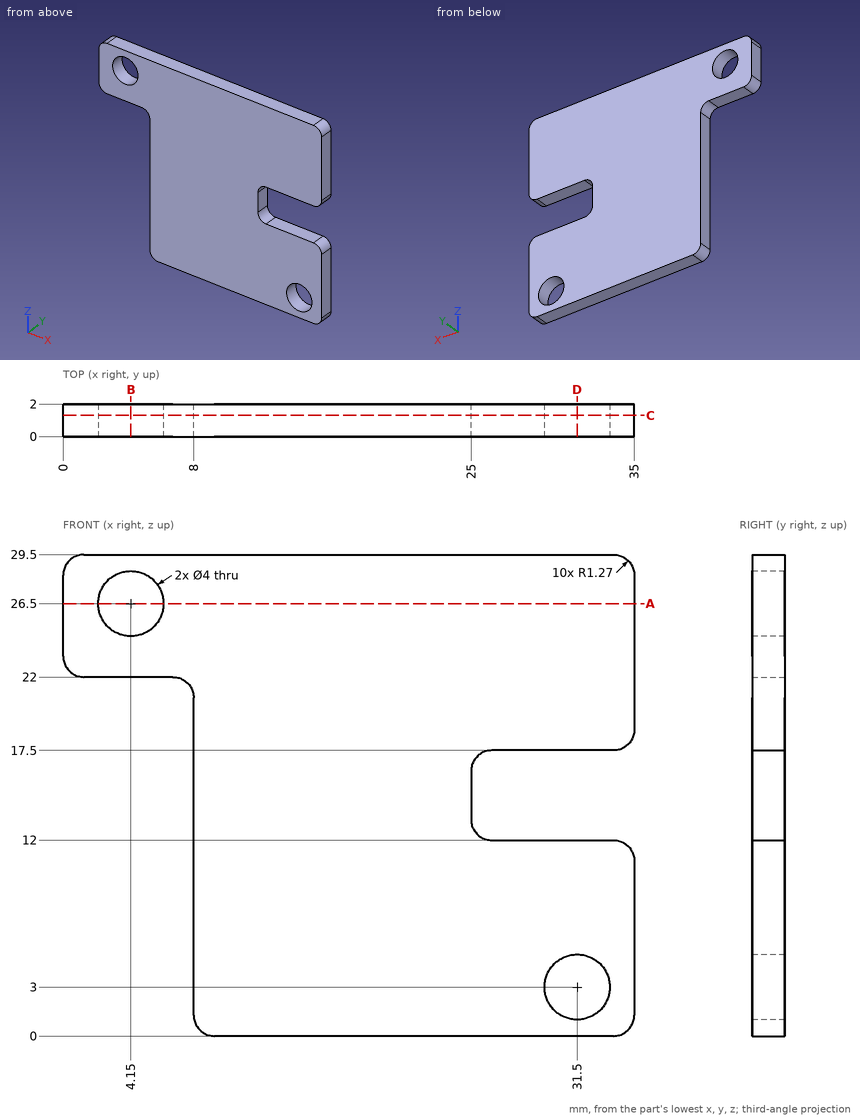
Can you work these out from the drawing? Everything is in mm from the part's minimum corner. Round coordinates to 2 decimals unless told otherwise and drop trailing zeros. Loops run counter-clockwise (first coordinate to the right, second up) from the corner with the lowest first, then second, coordinate; pieces in that order, holes last. Notation, with made-up numbers: (74.5, 46.5) - (91.5, 46.5) arc R5 cw to (91.5, 55.5) - close; hole circle Ø9 at (-27.75, 86.5). An arc over 180 degrees is marked (long way). Answer in a Markdown table with one row per item. Add a question column.
Q1. I want a section at A-A on z = 26.5. List the corners of the cut face in (x, y) for me, and give its area (3 significant figures).
Q2. I want a section at B-B on x = 4.15. List the corners of the cut face in (y, z) for me.
Q3. I need wall thicknesses on L1, parallel to X at y = 1.3, z = 26.5; L2, parallel to Z at x = 28.5, y = 0.9; L3, parallel to X at y = 1.55, z = 3. Which ranges of each line are inside material? Lowest first, please.
Q4. I want a section at C-C on y = 1.3. List the corners of the cut face in (x, z) for me, and give its area (3 significant figures).
Q5. I want a section at D-D on x = 31.5. List the corners of the cut face in (y, z) for me.
Q6. For pin 1 Ø0.6 at (x, y) = (4.5, 1.5) entering from -Z, with a flat end and sliding along its axis, tell me the tip position at first contact or that it passes through.
A:
| question | item | result |
|---|---|---|
| 1 | outline | (0, 0) - (2.15, 0) - (2.15, 2) - (0, 2) - close; (6.15, 0) - (35, 0) - (35, 2) - (6.15, 2) - close |
| 1 | area | 62.0 mm^2 |
| 2 | outline | (0, 22) - (2, 22) - (2, 24.5) - (0, 24.5) - close; (0, 28.5) - (2, 28.5) - (2, 29.5) - (0, 29.5) - close |
| 3 | L1 | 0 to 2.15, 6.15 to 35 |
| 3 | L2 | 0 to 12, 17.5 to 29.5 |
| 3 | L3 | 8 to 29.5, 33.5 to 35 |
| 4 | outline | (0, 23.27) arc R1.27 ccw to (1.27, 22) - (6.73, 22) arc R1.27 cw to (8, 20.73) - (8, 1.27) arc R1.27 ccw to (9.27, 0) - (33.73, 0) arc R1.27 ccw to (35, 1.27) - (35, 10.73) arc R1.27 ccw to (33.73, 12) - (26.27, 12) arc R1.27 cw to (25, 13.27) - (25, 16.23) arc R1.27 cw to (26.27, 17.5) - (33.73, 17.5) arc R1.27 ccw to (35, 18.77) - (35, 28.23) arc R1.27 ccw to (33.73, 29.5) - (1.27, 29.5) arc R1.27 ccw to (0, 28.23) - close; hole circle Ø4 at (4.15, 26.5); hole circle Ø4 at (31.5, 3) |
| 4 | area | 775 mm^2 |
| 5 | outline | (0, 0) - (2, 0) - (2, 1) - (0, 1) - close; (0, 5) - (2, 5) - (2, 12) - (0, 12) - close; (0, 17.5) - (2, 17.5) - (2, 29.5) - (0, 29.5) - close |
| 6 | pin 1 | z = 22 |
